Part model, mm, in its own coordinate system. Round coordinates to 2 decimals unless told otherwise and drop trailing zeros. Order: outer loops, then holes, each group sorted by start corner. A loop starts at its lowest first (then second) coordinate and runs counter-clockwise, first axis right, second up. Notation, with made-up numbers: (61, 8.25) - (113, 8.25) arc R32 cw to (113, 39.25) - close; hole circle Ø9 at (4, 89). An arc over 180 degrees is marked (long way). Answer as a JSON object with one key per item and string values.
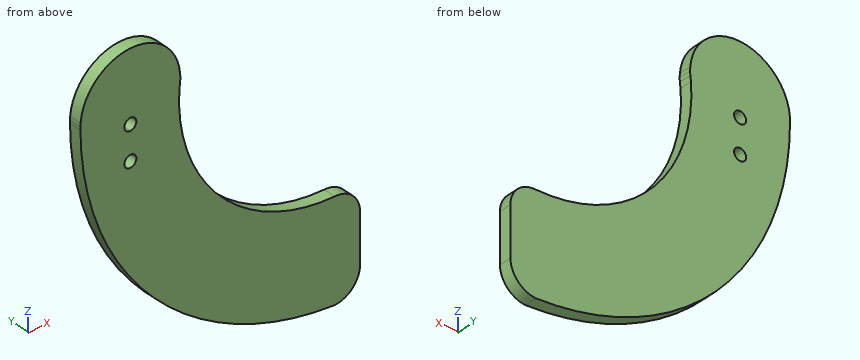
```python
from build123d import *

# Parameters (mm, degrees)
F0_R     = 1.5
F1_DEPTH = 3
F3_DEPTH = 381


with BuildPart() as f1:
    # F0 (on Front) → F1 (new body)
    with BuildSketch(Plane.XZ):
        with BuildLine():
            ThreePointArc((12.4599357944, -0.3280291537), (12.4796291372, -0.163973202), (12.5, 0))
            ThreePointArc((12.5, 0), (12.4899799325, 0.5004011242), (12.4599357944, 1))
            Line((12.4599357944, 1), (12.4599357944, -0.3280291537))
        make_face()
        with BuildLine():
            ThreePointArc((12.4599357944, -1), (12.4899799325, -0.5004011242), (12.5, 0))
            ThreePointArc((12.5, 0), (12.4796291372, -0.163973202), (12.4599357944, -0.3280291537))
            Line((12.4599357944, -0.3280291537), (12.4599357944, -1))
        make_face()
        with BuildLine():
            Line((12.4599357944, -0.3280291537), (12.4599357944, 1))
            ThreePointArc((12.4599357944, 1), (0, 12.5), (-12.4599357944, 1))
            Line((-12.4599357944, 1), (-12.4599357944, -1))
            ThreePointArc((-12.4599357944, -1), (-0.696307501, -12.4805911664), (12.2713731569, -2.3797900839))
            ThreePointArc((12.2713731569, -2.3797900839), (12.3524414608, -1.3526953053), (12.4599357944, -0.3280291537))
        make_face()
        Circle(F0_R, mode=Mode.SUBTRACT)
        with BuildLine():
            ThreePointArc((12.2713731569, -2.3797900839), (12.3848845687, -1.6925230338), (12.4599357944, -1))
            Line((12.4599357944, -1), (12.4599357944, -0.3280291537))
            ThreePointArc((12.4599357944, -0.3280291537), (12.3524414608, -1.3526953053), (12.2713731569, -2.3797900839))
        make_face()
        with BuildLine():
            Line((-12.4599357944, -1), (-12.4599357944, 1))
            ThreePointArc((-12.4599357944, 1), (-12.4899799325, 0.5004011242), (-12.5, 0))
            ThreePointArc((-12.5, 0), (-12.4899799325, -0.5004011242), (-12.4599357944, -1))
        make_face()
        with BuildLine():
            ThreePointArc((51.15, -45), (22.6329157643, -31.9707379741), (12.2713731569, -2.3797900839))
            ThreePointArc((12.2713731569, -2.3797900839), (-0.696307501, -12.4805911664), (-12.4599357944, -1))
            ThreePointArc((-12.4599357944, -1), (-12.4899799325, -0.5004011242), (-12.5, 0))
            Line((-12.5, 0), (-12.5, -0.5771173286))
            ThreePointArc((-12.5, -0.5771173286), (5.9031905044, -47.5942731711), (51.15, -70))
            ThreePointArc((51.15, -70), (55.6401280605, -68.1401280605), (57.5, -63.65))
            Line((57.5, -63.65), (57.5, -51.35))
            ThreePointArc((57.5, -51.35), (55.6401280605, -46.8598719395), (51.15, -45))
        make_face()
        with BuildLine():
            Line((-12.5, -0.5771173286), (-12.5, 0))
            ThreePointArc((-12.5, 0), (-12.5005947604, -0.2885586643), (-12.5, -0.5771173286))
        make_face()
        Circle(F0_R)
    extrude(amount=F1_DEPTH)

    # F2 (on face) → F3 (cut, symmetric)
    with BuildSketch(Plane.XZ.offset(3)):
        with BuildLine():
            ThreePointArc((1.5, -5), (1.0606601718, -3.9393398282), (0, -3.5))
            Line((0, -3.5), (0, -5))
            Line((0, -5), (0, -6.5))
            ThreePointArc((0, -6.5), (1.0606601718, -6.0606601718), (1.5, -5))
        make_face()
        with BuildLine():
            ThreePointArc((1.5, -13.5), (1.0606601718, -12.4393398282), (0, -12))
            ThreePointArc((0, -12), (-1.0606601718, -14.5606601718), (1.5, -13.5))
        make_face()
        with BuildLine():
            Line((0, -5), (0, -3.5))
            ThreePointArc((0, -3.5), (-1.5, -5), (0, -6.5))
            Line((0, -6.5), (0, -5))
        make_face()
    extrude(amount=F3_DEPTH, both=True, mode=Mode.SUBTRACT)


solid = f1.part
```
Item 1: Drop a flat-ended pin along its axis: P1, Ø1, axis at y = -2, z = -17.5, coming from the -X side. Give the stop position or say it passes through.
Taken from the geometry:
{"P1": "x = -10.48"}
Item 2: Cut at A-A (y = -2.55). Write the cut outline in (x, z).
Taken from the geometry:
{"outline": "(-12.5, 0) arc R70 ccw to (51.15, -70) arc R6.35 ccw to (57.5, -63.65) - (57.5, -51.35) arc R6.35 ccw to (51.15, -45) arc R40 cw to (12.27, -2.38) arc R12.5 ccw (long way) to start; hole circle Ø3 at (0, -13.5); hole circle Ø3 at (0, -5)"}
Item 3: Cut at B-B (z = -54). Write the cut outline in (x, y), plus the area to 3 significant figures.
Taken from the geometry:
{"outline": "(12.61, -3) - (57.5, -3) - (57.5, 0) - (12.61, 0) - close", "area": "135 mm2"}
Item 4: Cut at C-C (x = 8.5). Write the cut outline in (y, z), plus the area to 3 significant figures.
Taken from the geometry:
{"outline": "(-3, -50.28) - (0, -50.28) - (0, 9.17) - (-3, 9.17) - close", "area": "178 mm2"}
Item 5: Probe L1, parallel to X at y = -0.75, z = -12.5; L2, parallel to X at y = -2, z = -13.5; L3, parallel to Z at x = 51, y = -1. List the from-to ranges inside material, lowest first. Write a range as from..to.
Taken from the geometry:
{"L1": "-11.43..-1.12, 1.12..12.89", "L2": "-11.24..-1.5, 1.5..13.1", "L3": "-69.99..-45"}
